```python
from build123d import *

# Parameters (mm, degrees)
F0_W     = 71.266532
F0_H     = 49.356132
F1_DEPTH = 25.4
F2_R     = 10.06801
F3_DEPTH = 25.4
F5_DEPTH = 46.228


with BuildPart() as f1:
    # F0 (on Top) → F1 (new body)
    with BuildSketch(Plane.XY):
        Rectangle(F0_W, F0_H)
    extrude(amount=F1_DEPTH)

    # F2 (on face) → F3 (join)
    with BuildSketch(Plane.XY.offset(25.4)):
        Circle(F2_R)
    extrude(amount=F3_DEPTH)

    # F4 (on face) → F5 (cut)
    with BuildSketch(Plane.XZ.offset(24.678066)):
        Polygon((15.782516, 50.946049), (-10.0584, 50.946049), (15.782516, 31.35702), align=None)
    extrude(amount=-F5_DEPTH, mode=Mode.SUBTRACT)


solid = f1.part
```
Work out the finished part from the listing and answer in its coordinate system (mm). A direction names the side the tool comes from. Coordinates: 2 decimals unless noted, no trailing zeros. Loops run counter-clockwise (first coordinate to the right, second up) from the corner with the lowest first, then second, coordinate; pieces in that order, holes last.
1) Section C-C (z = 29) is taken. Give the vertices of the cut face in (x, y).
Results:
outline: circle Ø20.14 at (0, 0)
2) Flat-ended cylindrical pins translate along their axes: pin 1 (15 mm diameter, centred on x = 14.5, y = -12, fed in from +Z); pin 2 (6 mm diameter, centred on y = -15.5, z = 42, fed in from -X); pin 3 (12 mm diameter, centred on y = -14, z = 31.5, fed in from +X); pin 4 (5 mm diameter, centred on x = 8.5, z = 29.5, fed in from +Y). Find the tip coordinate at first contact, or state that the pin passes through.
Results:
pin 1: stops at z = 25.4
pin 2: passes through
pin 3: stops at x = 6.11
pin 4: stops at y = 8.08
3) Section B-B (x = 0) is taken. Give the vertices of the cut face in (y, z), plus the area to 3 significant figures.
Results:
outline: (-24.68, 0) - (24.68, 0) - (24.68, 25.4) - (10.07, 25.4) - (10.07, 43.32) - (-10.07, 43.32) - (-10.07, 25.4) - (-24.68, 25.4) - close
area: 1,610 mm2
4) Section D-D (x = 31.5) is taken. Give the vertices of the cut face in (y, z), plus the area to 3 significant figures.
Results:
outline: (-24.68, 0) - (24.68, 0) - (24.68, 25.4) - (-24.68, 25.4) - close
area: 1,250 mm2
5) Section A-A (y = 0) is taken. Give the vertices of the cut face in (x, z), plus the area to 3 significant figures.
Results:
outline: (-35.63, 0) - (35.63, 0) - (35.63, 25.4) - (10.07, 25.4) - (10.07, 35.69) - (-9.87, 50.8) - (-10.07, 50.8) - (-10.07, 25.4) - (-35.63, 25.4) - close
area: 2,170 mm2
6) Consider probe 1 along Z at (x, y) = (19.5, 19); probe 2 along Y at (x, z) = (5, 35); probe 3 along Z at (x, y) = (-5, 2). Determine where each line is inside the solid, lowest interval first.
Results:
probe 1: z = 0 to 25.4
probe 2: y = -8.74 to 8.74
probe 3: z = 0 to 47.11
7) For faces 1 (the flat face through (35.633, 0, 13)), 2 (the flat face through (-8.42, 5.83, 25.4)), determine the directions among +Z, -Z, +X, -X, +Y, -Y from which every point of the face is accessible in a straight line to the end or side of a thin tool.
Results:
face 1: +Z, -Z, +X, +Y, -Y
face 2: +Z
